```python
from build123d import *

# Parameters (mm, degrees)
SKETCH1_R           = 3.25
BOSS_EXTRUDE1_DEPTH = 3
CUT_EXTRUDE1_REACH  = 124.855
SKETCH2_W           = 30
SKETCH2_H           = 1.5


with BuildPart() as part:
    # Sketch1 → Boss-Extrude1 (new body)
    with BuildSketch(Plane.XY):
        Polygon((-27.792893219, 25), (-45.5, 25), (-72.207106781, 25), (-77.5, 30.292893219), (-77.5, 69.792893219), (-80.207106781, 72.5), (-96.792893219, 72.5), (-99.5, 69.792893219), (-99.5, 3.207106781), (-96.792893219, 0.5), (-50.760240095, 0.5), (-3.207106781, 0.5), (-0.5, 3.207106781), (-0.5, 69.792893219), (-3.207106781, 72.5), (-19.792893219, 72.5), (-22.5, 69.792893219), (-22.5, 30.292893219), align=None)
        with Locations((-6.5, 66.5)):
            Circle(SKETCH1_R, mode=Mode.SUBTRACT)
        with Locations((-6.5, 6.5)):
            Circle(SKETCH1_R, mode=Mode.SUBTRACT)
        with Locations((-93.5, 6.5)):
            Circle(SKETCH1_R, mode=Mode.SUBTRACT)
        with Locations((-93.5, 66.5)):
            Circle(SKETCH1_R, mode=Mode.SUBTRACT)
    extrude(amount=BOSS_EXTRUDE1_DEPTH)

    # Sketch2 → Cut-Extrude1 (cut, up to next)
    with BuildSketch(Plane.XZ.offset(-0.5), mode=Mode.PRIVATE) as cut_extrude1_sk1:
        with Locations((-50, 1.5)):
            Rectangle(SKETCH2_W, SKETCH2_H)
    cut_extrude1_tool1 = extrude(cut_extrude1_sk1.sketch, amount=-CUT_EXTRUDE1_REACH, mode=Mode.PRIVATE) & part.part
    add(cut_extrude1_tool1.solids().sort_by_distance((-50, 0.5, 1.5))[0], mode=Mode.SUBTRACT)


solid = part.part
```
Read the model definition and answer for the solid it produces. Units are mm, in the model's axes. A direction names the side the tool comes from. Round coordinates to 2 decimals unless told otherwise and drop trailing zeros. Loops run counter-clockwise (first coordinate to the right, second up) from the corner with the lowest first, then second, coordinate; pieces in that order, holes last. Notation, with made-up numbers: (5.25, 19) -> (20.25, 19) arc R16 ccw to (20.25, 26) -> close; hole circle Ø4 at (-15, 5). An arc over 180 degrees is marked (long way). One line per item, written item: value.
1) For faces 4 (the face through (-25.109, 27.683, 1.479)), 5 (the face through (-96.079, 64.522, 1.479)), 6 (the face through (-50, 13, 0.75)), determine the directions among +Z, -Z, +X, -X, +Y, -Y from which every point of the face is accessible in a straight line to the end or side of a thin tool.
Answer list:
face 4: +Z, -Z, +Y
face 5: +Z, -Z
face 6: +Y, -Y
2) A cutting plane is placed at D-D (x = -36.5). Determine the outline of the cut face in (y, z).
Answer list:
outline: (0.5, 0) -> (25, 0) -> (25, 0.75) -> (0.5, 0.75) -> close; (0.5, 2.25) -> (25, 2.25) -> (25, 3) -> (0.5, 3) -> close
3) Consider L1, parallel to Y at x = -6.5, z = 2.25; L2, parallel to Z at x = -46.5, y = 14.5; L3, parallel to X at y = 41.5, z = 0.1. Determine where each line is inside the solid, lowest interval first. Write a range as [from, to].
Answer list:
L1: y = [0.5, 3.25], [9.75, 63.25], [69.75, 72.5]
L2: z = [0, 0.75], [2.25, 3]
L3: x = [-99.5, -77.5], [-22.5, -0.5]
4) A cutting plane is placed at A-A (y = 54.5). Determine the outline of the cut face in (x, z), and give its area (3 significant figures).
Answer list:
outline: (-99.5, 0) -> (-77.5, 0) -> (-77.5, 3) -> (-99.5, 3) -> close; (-22.5, 0) -> (-0.5, 0) -> (-0.5, 3) -> (-22.5, 3) -> close
area: 132 mm²
5) A cutting plane is placed at B-B (x = -6.5). Determine the outline of the cut face in (y, z).
Answer list:
outline: (0.5, 0) -> (3.25, 0) -> (3.25, 3) -> (0.5, 3) -> close; (9.75, 0) -> (63.25, 0) -> (63.25, 3) -> (9.75, 3) -> close; (69.75, 0) -> (72.5, 0) -> (72.5, 3) -> (69.75, 3) -> close
6) The mould has two halves that part along Y. Classify faces 1 (the face through (-1.835, 71.127, 1.479)), 2 (the face through (-77.5, 50, 1)), 3 (the face through (-4.75, 9.24, 1.48)): pulls with the +Y half, pulls with the -Y half, needs draft (parallel to the pull), parting line crosses it, or undercut.
Answer list:
face 1: pulls with the +Y half
face 2: needs draft
face 3: undercut
7) A cutting plane is placed at C-C (y = 6.5). Determine the outline of the cut face in (x, z).
Answer list:
outline: (-99.5, 0) -> (-96.75, 0) -> (-96.75, 3) -> (-99.5, 3) -> close; (-90.25, 0) -> (-9.75, 0) -> (-9.75, 3) -> (-90.25, 3) -> close; (-3.25, 0) -> (-0.5, 0) -> (-0.5, 3) -> (-3.25, 3) -> close; hole (-65, 0.75) -> (-35, 0.75) -> (-35, 2.25) -> (-65, 2.25) -> close
